from build123d import *

# Parameters (mm, degrees)
SKETCH1_R           = 2.54
SKETCH1_R_2         = 4.7625
BOSS_EXTRUDE1_DEPTH = 36.068


with BuildPart() as part:
    # Sketch1 → Boss-Extrude1 (new body)
    with BuildSketch(Plane.XY):
        with BuildLine():
            Line((65.395995047, 51.923287663), (57.425031933, 75.072645444))
            ThreePointArc((57.425031933, 75.072645444), (56.26674234, 76.623783324), (54.423010456, 77.213966553))
            Line((54.423010456, 77.213966553), (-17.406388387, 77.213966553))
            ThreePointArc((-17.406388387, 77.213966553), (-19.250120272, 76.623783324), (-20.408409865, 75.072645444))
            Line((-20.408409865, 75.072645444), (-28.379372979, 51.923287663))
            Line((-28.379372979, 51.923287663), (-28.379372979, -5.244694556))
            Line((-28.379372979, -5.244694556), (-20.408409865, -28.394052337))
            ThreePointArc((-20.408409865, -28.394052337), (-19.250120272, -29.945190218), (-17.406388387, -30.535373447))
            Line((-17.406388387, -30.535373447), (54.423010456, -30.535373447))
            ThreePointArc((54.423010456, -30.535373447), (56.26674234, -29.945190218), (57.425031933, -28.394052337))
            Line((57.425031933, -28.394052337), (65.395995047, -5.244694556))
            Line((65.395995047, -5.244694556), (65.395995047, 51.923287663))
        make_face()
        with Locations((-13.241688966, 67.785486553)):
            Circle(SKETCH1_R, mode=Mode.SUBTRACT)
        with Locations((50.258311034, 67.785486553)):
            Circle(SKETCH1_R, mode=Mode.SUBTRACT)
        with Locations((-20.137788966, -21.106893447)):
            Circle(SKETCH1_R, mode=Mode.SUBTRACT)
        with Locations((57.154411034, -21.106893447)):
            Circle(SKETCH1_R, mode=Mode.SUBTRACT)
        with Locations((-20.215986176, 25.397966553)):
            Circle(SKETCH1_R_2, mode=Mode.SUBTRACT)
        with Locations((57.232608244, 25.397966553)):
            Circle(SKETCH1_R_2, mode=Mode.SUBTRACT)
    extrude(amount=BOSS_EXTRUDE1_DEPTH)


solid = part.part
Can you work these out from the model? Positions are in its coordinate system, mm. Give positions to 0.01 mm unless a question says otherwise; leave off trailing zeros. Return JSON: item names as keys, results as strings.
Q1. I want a section at A-A, the plane z = 29.5. Count the separate pieces of the cut face and the enclosed holes in it, then the cut area to 3 significant figures.
Checks:
{"separate pieces": "1", "enclosed holes": "6", "area": "9,440 mm2"}
Q2. For pin 1 Ø8 at (y, z) = (-17, 25) entering from -X; pin 2 Ø8.5 at (x, y) = (57.23, 25.4) entering from +Z; pin 3 Ø6 at (y, z) = (61, 9.5) entering from +X, each with a flat end and sliding along its axis, tell me the tip position at first contact or that it passes through.
Checks:
{"pin 1": "stops at x = -25.71", "pin 2": "passes through", "pin 3": "stops at x = 63.3"}
Q3. I need wall thicknesses on probe 1 along X at (y, z) = (67, 34.5); probe 2 along X at (y, z) = (-19, 11.5); probe 3 along Y at (x, z) = (53.5, 32.5). Which ranges of each line are inside material? Lowest first, please.
Checks:
{"probe 1": "x = -23.19 to -15.66, -10.83 to 47.84, 52.67 to 60.2", "probe 2": "x = -23.64 to -21.56, -18.72 to 55.74, 58.57 to 60.66", "probe 3": "y = -30.54 to 22.44, 28.36 to 77.21"}
Q4. We'd pull the mould along Y, two halves only. Please class faces 1 (the face through (-20.47, -18.59, 17.78)), 2 (the face through (18, 24, 0)), 3 (the face through (19, 77.214, 18)): released by +Y, released by -Y, zero draft, split by the parting line, or undercut.
Checks:
{"face 1": "undercut", "face 2": "zero draft", "face 3": "released by +Y"}
